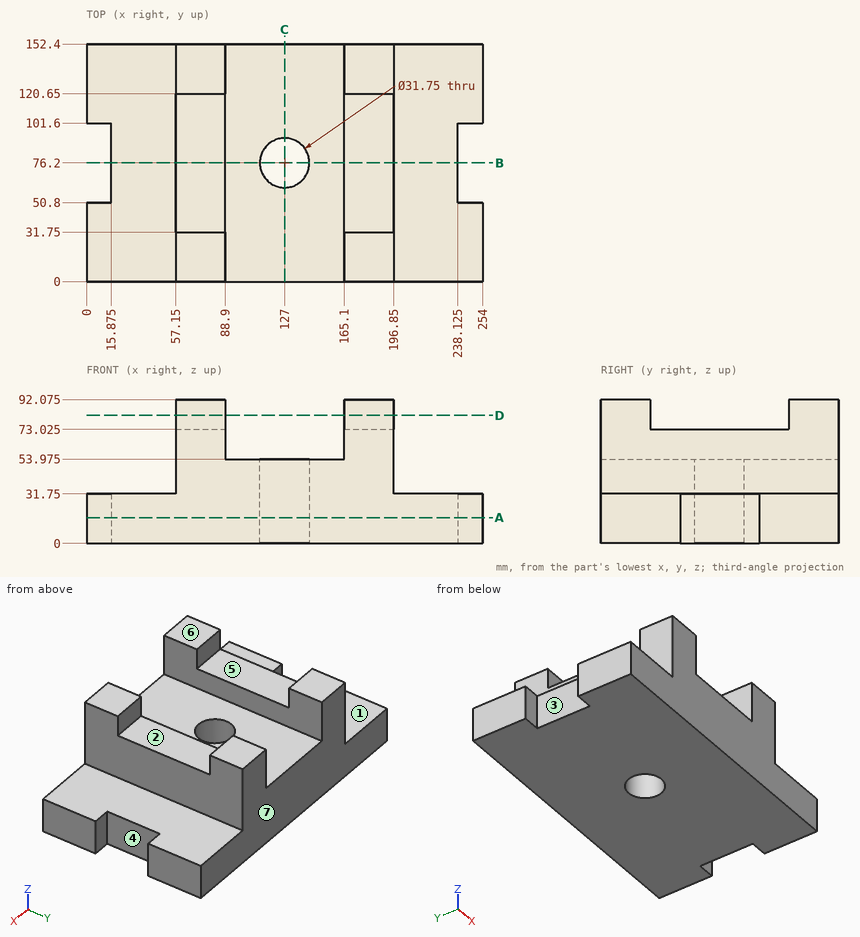
Here's the drawing with two shaded views (mm, measured from the low corner). I have some questions. A direction names the side the tool comes from. Coordinates: 2 decimals unless noted, no trailing zeros. Write each loop counter-clockwise with the first axis right and the second up, starting at its lowest first coordinate (ties: lowest second). Pieces come first, ordered by that corner, then holes. Notation, with made-up numbers: (-3.75, -23) -> (51.25, -23) arc R27 ccw to (51.25, -5) -> close; hole circle Ø8 at (-10.5, -20). An arc over 180 degrees is marked (long way). Answer as CSV lines item,"result".
1) If we section it at A-A on z = 16.5: Please give me the cut outline in (x, y) (3 decimals), then the cut area to 3 significant figures.
Check result:
outline,"(0, 0) -> (254, 0) -> (254, 50.8) -> (238.125, 50.8) -> (238.125, 101.6) -> (254, 101.6) -> (254, 152.4) -> (0, 152.4) -> (0, 101.6) -> (15.875, 101.6) -> (15.875, 50.8) -> (0, 50.8) -> close; hole circle Ø31.75 at (127, 76.2)"
area,"36,300 mm²"
2) If we section it at C-C on x = 127: Please give me the cut outline in (y, z) (3 decimals).
Check result:
outline,"(0, 0) -> (60.325, 0) -> (60.325, 53.975) -> (0, 53.975) -> close; (92.075, 0) -> (152.4, 0) -> (152.4, 53.975) -> (92.075, 53.975) -> close"
3) On a 3-axis mill with a long thin cutter (end or side, diameter ignored), from which of +Z, -Z, +X, -X, +Y, -Y can I reach the whole of each face in a straight line? I mean the marked faces 1, 2, 3 and 4. Say none if no direction works.
Check result:
face 1,"+Z, -X, +Y, -Y"
face 2,"+Z, +X, -X"
face 3,"+Z, -Z, -X"
face 4,"+Z, -Z, +X"
4) If we section it at D-D on z = 82: Please give me the cut outline in (x, y), then the cut area to 3 significant figures.
Check result:
outline,"(57.15, 0) -> (88.9, 0) -> (88.9, 31.75) -> (57.15, 31.75) -> close; (57.15, 120.65) -> (88.9, 120.65) -> (88.9, 152.4) -> (57.15, 152.4) -> close; (165.1, 0) -> (196.85, 0) -> (196.85, 31.75) -> (165.1, 31.75) -> close; (165.1, 120.65) -> (196.85, 120.65) -> (196.85, 152.4) -> (165.1, 152.4) -> close"
area,"4,030 mm²"
5) If we section it at B-B on y = 76.2: Please give me the cut outline in (x, z) (3 decimals), then the cut area to 3 significant figures.
Check result:
outline,"(15.875, 0) -> (111.125, 0) -> (111.125, 53.975) -> (88.9, 53.975) -> (88.9, 73.025) -> (57.15, 73.025) -> (57.15, 31.75) -> (15.875, 31.75) -> close; (142.875, 0) -> (238.125, 0) -> (238.125, 31.75) -> (196.85, 31.75) -> (196.85, 73.025) -> (165.1, 73.025) -> (165.1, 53.975) -> (142.875, 53.975) -> close"
area,"9,660 mm²"
6) Will these pins go through, and if not, where does the flat tip stop? P1, Ø1, axis at y = 45.5, z = 50, coming from the -X side; P2, Ø9.5, axis at y = 81, z = 19, coming from the +X side (3 decimals); P3, Ø9.5, axis at x = 182.5, y = 70, coming from the +Z side (3 decimals).
Check result:
P1,"x = 57.15"
P2,"x = 238.125"
P3,"z = 73.025"
7) If I drill on line 1 (X direction, y = 76, z = 35); line 2 (X direction, y = 23, z = 64); line 3 (Y direction, x = 127, z = 21) (3 decimals), over which ranges is the centre line in solid material (lowest first)? Write a range as from..to.
Check result:
line 1,"57.15..111.13, 142.87..196.85"
line 2,"57.15..88.9, 165.1..196.85"
line 3,"0..60.325, 92.075..152.4"
8) If we mould it in two halves opening along Y, with no side actions, what happens to the marked faces 5, 6 and 7? For each: +Y half, -Y half, draft (parallel to the pull), parting line (faces both ways), or undercut.
Check result:
face 5,"undercut"
face 6,"draft"
face 7,"+Y half"
